Here's how the part is built. I have some questions about the finished solid (model axes, mm). Round coordinates to 2 decimals unless told otherwise and drop trailing zeros.
Autodesk Inventor part; units mm, degrees
ref_plane "C1_XY" through (0, 0, 0) normal (0, 0, 1) x (1, 0, 0)
ref_plane "C1_YZ" through (0, 0, 0) normal (1, 0, 0) x (0, 1, 0)
ref_plane "C1_ZX" through (0, 0, 0) normal (0, 1, 0) x (0, 0, 1)
sketch "Sketch_1" plane through (0, 0, 0) normal (0, 0, 1) x (1, 0, 0)
  line L0 (-10, -7) -> (-8, -7)
  line L1 (-8, -7) -> (-8, -4)
  line L2 (-8, -4) -> (-7.0607, -4)
  line L3 (-7.0607, -4) -> (-4, -7.0607)
  line L4 (-4, -7.0607) -> (-4, -9.4804)
  line L5 (-4, -9.4804) -> (-3.7, -10)
  line L6 (-3.7, -10) -> (-4, -10.5196)
  line L7 (-4, -10.5196) -> (-4, -12.9393)
  line L8 (-4, -12.9393) -> (-7.0607, -16)
  line L9 (-7.0607, -16) -> (-8, -16)
  line L10 (-8, -16) -> (-8, -13)
  line L11 (-8, -13) -> (-10, -13)
  line L12 (-10, -13) -> (-10, -19)
  arc A0 (-10, -19) -> (-9, -20) centre (-9, -19) ccw
  line L13 (-9, -20) -> (-3, -20)
  line L14 (-3, -20) -> (-3, -18)
  line L15 (-3, -18) -> (-6, -18)
  line L16 (-6, -18) -> (-6, -17.0607)
  line L17 (-6, -17.0607) -> (-2.9393, -14)
  line L18 (-2.9393, -14) -> (-0.5196, -14)
  line L19 (-0.5196, -14) -> (0, -13.7)
  line L20 (0, -13.7) -> (0.5196, -14)
  line L21 (0.5196, -14) -> (2.9393, -14)
  line L22 (2.9393, -14) -> (6, -17.0607)
  line L23 (6, -17.0607) -> (6, -18)
  line L24 (6, -18) -> (3, -18)
  line L25 (3, -18) -> (3, -20)
  line L26 (3, -20) -> (9, -20)
  arc A1 (9, -20) -> (10, -19) centre (9, -19) ccw
  line L27 (10, -19) -> (10, -13)
  line L28 (10, -13) -> (8, -13)
  line L29 (8, -13) -> (8, -16)
  line L30 (8, -16) -> (7.0607, -16)
  line L31 (7.0607, -16) -> (4, -12.9393)
  line L32 (4, -12.9393) -> (4, -10.5196)
  line L33 (4, -10.5196) -> (3.7, -10)
  line L34 (3.7, -10) -> (4, -9.4804)
  line L35 (4, -9.4804) -> (4, -7.0607)
  line L36 (4, -7.0607) -> (7.0607, -4)
  line L37 (7.0607, -4) -> (8, -4)
  line L38 (8, -4) -> (8, -7)
  line L39 (8, -7) -> (10, -7)
  line L40 (10, -7) -> (10, 7)
  line L41 (10, 7) -> (8, 7)
  line L42 (8, 7) -> (8, 4)
  line L43 (8, 4) -> (7.0607, 4)
  line L44 (7.0607, 4) -> (4, 7.0607)
  line L45 (4, 7.0607) -> (4, 9.4804)
  line L46 (4, 9.4804) -> (3.7, 10)
  line L47 (3.7, 10) -> (4, 10.5196)
  line L48 (4, 10.5196) -> (4, 12.9393)
  line L49 (4, 12.9393) -> (7.0607, 16)
  line L50 (7.0607, 16) -> (8, 16)
  line L51 (8, 16) -> (8, 13)
  line L52 (8, 13) -> (10, 13)
  line L53 (10, 13) -> (10, 19)
  arc A2 (10, 19) -> (9, 20) centre (9, 19) ccw
  line L54 (9, 20) -> (3, 20)
  line L55 (3, 20) -> (3, 18)
  line L56 (3, 18) -> (6, 18)
  line L57 (6, 18) -> (6, 17.0607)
  line L58 (6, 17.0607) -> (2.9393, 14)
  line L59 (2.9393, 14) -> (0.5196, 14)
  line L60 (0.5196, 14) -> (0, 13.7)
  line L61 (0, 13.7) -> (-0.5196, 14)
  line L62 (-0.5196, 14) -> (-2.9393, 14)
  line L63 (-2.9393, 14) -> (-6, 17.0607)
  line L64 (-6, 17.0607) -> (-6, 18)
  line L65 (-6, 18) -> (-3, 18)
  line L66 (-3, 18) -> (-3, 20)
  line L67 (-3, 20) -> (-9, 20)
  arc A3 (-9, 20) -> (-10, 19) centre (-9, 19) ccw
  line L68 (-10, 19) -> (-10, 13)
  line L69 (-10, 13) -> (-8, 13)
  line L70 (-8, 13) -> (-8, 16)
  line L71 (-8, 16) -> (-7.0607, 16)
  line L72 (-7.0607, 16) -> (-4, 12.9393)
  line L73 (-4, 12.9393) -> (-4, 10.5196)
  line L74 (-4, 10.5196) -> (-3.7, 10)
  line L75 (-3.7, 10) -> (-4, 9.4804)
  line L76 (-4, 9.4804) -> (-4, 7.0607)
  line L77 (-4, 7.0607) -> (-7.0607, 4)
  line L78 (-7.0607, 4) -> (-8, 4)
  line L79 (-8, 4) -> (-8, 7)
  line L80 (-8, 7) -> (-10, 7)
  line L81 (-10, 7) -> (-10, -7)
  line L82 (-8, 1.7) -> (-8, -1.7)
  arc A4 (-8, -1.7) -> (-7.7, -2) centre (-7.7, -1.7) ccw
  line L83 (-7.7, -2) -> (-7.0636, -2)
  arc A5 (-6.8515, -2.0879) -> (-7.0636, -2) centre (-7.0636, -2.3) ccw
  line L84 (-6.8515, -2.0879) -> (-2.9393, -6)
  line L85 (-2.9393, -6) -> (2.9393, -6)
  line L86 (2.9393, -6) -> (6.8515, -2.0879)
  arc A6 (7.0636, -2) -> (6.8515, -2.0879) centre (7.0636, -2.3) ccw
  line L87 (7.0636, -2) -> (7.7, -2)
  arc A7 (7.7, -2) -> (8, -1.7) centre (7.7, -1.7) ccw
  line L88 (8, -1.7) -> (8, 1.7)
  arc A8 (8, 1.7) -> (7.7, 2) centre (7.7, 1.7) ccw
  line L89 (7.7, 2) -> (7.0636, 2)
  arc A9 (6.8515, 2.0879) -> (7.0636, 2) centre (7.0636, 2.3) ccw
  line L90 (6.8515, 2.0879) -> (2.9393, 6)
  line L91 (2.9393, 6) -> (-2.9393, 6)
  line L92 (-2.9393, 6) -> (-6.8515, 2.0879)
  arc A10 (-7.0636, 2) -> (-6.8515, 2.0879) centre (-7.0636, 2.3) ccw
  line L93 (-7.0636, 2) -> (-7.7, 2)
  arc A11 (-7.7, 2) -> (-8, 1.7) centre (-7.7, 1.7) ccw
extrude "Extrusion1" add sketch "Sketch_1" against normal blind 600
sketch "Sketch2" plane through (0, 0, -600) normal (0, 0, -1) x (-1, 0, 0)
  point P0 (0, 10)
hole "Hole1" at (0, 10, -600) direction (0, 0, 1) diameter 4.2 depth 600
pattern_linear "Rectangular Pattern1" count 2 spacing 20 along (0, -1, 0) of "Hole1"
ref_plane "C1_XY" through (0, 0, 0) normal (0, 0, 1) x (1, 0, 0)
ref_plane "C1_YZ" through (0, 0, 0) normal (1, 0, 0) x (0, 1, 0)
ref_plane "C1_ZX" through (0, 0, 0) normal (0, 1, 0) x (0, 0, 1)
properties part number "HFS5-2040-600"
1. If we section it at A-A, the plane z = -550: State how many separate pieces and enclosed holes the cut face has, and give its area (3 significant figures).
Evaluation:
separate pieces: 1
enclosed holes: 3
area: 324 mm2
2. I'm going to push flat-ended pins straight in: P1, Ø1.9, axis at y = -8.5, z = -222, coming from the +X side; P2, Ø0.6, axis at y = 19.5, z = -294, coming from the +X side; P3, Ø1.9, axis at x = 1, z = -327.5, coming from the +Y side. Where does each tip first touch, or does it pass through?
Evaluation:
P1: stops at x = 4
P2: stops at x = 9.98
P3: stops at y = 14
3. I need wall thicknesses on probe 1 along Y at (x, z) = (0, -139); probe 2 along X at (y, z) = (15, -417); probe 3 along Y at (x, z) = (-5, -421). Which ranges of each line are inside material? Lowest first, please.
Evaluation:
probe 1: y = -13.7 to -12.1, -7.9 to -6, 6 to 7.9, 12.1 to 13.7
probe 2: x = -10 to -8, -6.06 to -3.94, 3.94 to 6.06, 8 to 10
probe 3: y = -20 to -18, -16.06 to -13.94, -6.06 to -3.94, 3.94 to 6.06, 13.94 to 16.06, 18 to 20
